```python
from build123d import *

# Parameters (mm, degrees)
F1_DEPTH = 53.975
F3_DEPTH = 130.176


with BuildPart() as f1:
    # F0 (on Front) → F1 (new body)
    with BuildSketch(Plane.XZ):
        Polygon((-130.175, 0), (0, 0), (0, 21.8301708018), (-5.5739317977, 25.0482818256), (-66.675, 60.325), (-130.175, 60.325), align=None)
    extrude(amount=F1_DEPTH)

    # F2 (on face) → F3 (cut, through all)
    with BuildSketch(Plane(origin=(-130.175, 0, 0), x_dir=(0, -1, 0), z_dir=(-1, 0, 0))):
        Polygon((31.7433195945, 60.325), (53.975, 21.8186), (53.975, 60.325), align=None)
    extrude(amount=-F3_DEPTH, mode=Mode.SUBTRACT)


solid = f1.part
```
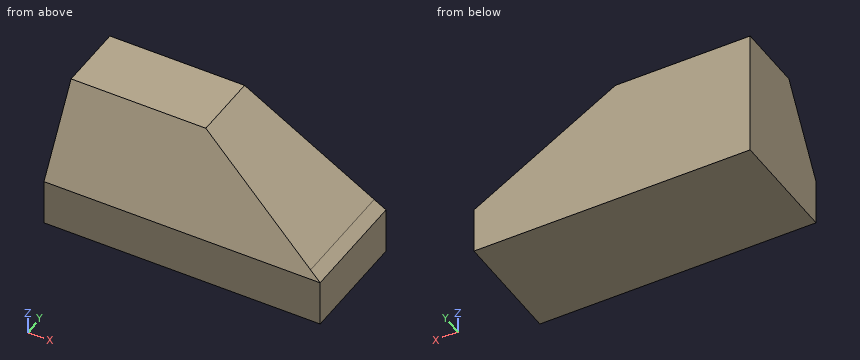
Model file for the job. Use its own axes, mm. Round coordinates to 2 decimals unless told otherwise and drop trailing zeros. Loops run counter-clockwise (first coordinate to the right, second up) from the corner with the lowest first, then second, coordinate; pieces in that order, holes last. Notation, with made-up numbers: M 86,-39.75 L 122,-39.75 A13 cw 122,-14.75 Z; hole C 53.25,26.25 d10. An arc over 180 degrees is marked long. Put each result on its own line as item: value. Start each with the question number.
Item 1: Drill centre lines: line 1 along Z through (x, y) = (-107.5, -33); line 2 along X through (y, z) = (-43.5, 39) (3 decimals); line 3 along X through (y, z) = (-19, 30.5) (3 decimals). Where is each one in solid material? Low to high.
Item 2: Drop flat-ended pins along their axis: P1, Ø10, axis at x = -105, z = 27.5, coming from the -Y side; P2, Ø1, axis at y = -5.5, z = 44.5, coming from the +X side; P3, Ø1.5, axis at y = -38, z = 43.5, coming from the +X side. Give the stop position or say it passes through.
Item 3: Cut at B-B (y = -21.5). List the corners of the cut face in (x, z) (3 decimals), then the cut area to 3 significant figures.
Item 4: Cut at D-D (x = -30). List the corners of the cut face in (y, z) (3 decimals).
Item 5: Cut at C-C (z = 49.5). List the corners of the cut face in (x, y) (3 decimals), then the cut area to 3 significant figures.
Item 6: Cut at A-A (x = -116). List the corners of the cut face in (y, z) (3 decimals), then the cut area to 3 significant figures.
Answer block:
1. line 1: 0 to 58.15
1. line 2: -130.175 to -29.739
1. line 3: -130.175 to -15.017
2. P1: y = -53.58
2. P2: x = -38.4
2. P3: x = -36.23
3. outline: M -130.175,0 L 0,0 L 0,21.83 L -66.675,60.325 L -130.175,60.325 Z
3. area: 6,570 mm2
4. outline: M -53.975,0 L 0,0 L 0,39.151 L -43.968,39.151 L -53.975,21.819 Z
5. outline: M -130.175,-37.993 L -47.926,-37.993 L -47.926,0 L -130.175,0 Z
5. area: 3,120 mm2
6. outline: M -53.975,0 L 0,0 L 0,60.325 L -31.743,60.325 L -53.975,21.819 Z
6. area: 2,830 mm2
